Geometry check sheet. Reference: the model listing, model coordinates, mm. Round coordinates to 2 decimals unless told otherwise and drop trailing zeros. Loops run counter-clockwise (first coordinate to the right, second up) from the corner with the lowest first, then second, coordinate; pieces in that order, holes last. Notation, with made-up numbers: (66.25, 53.5) - (122.25, 53.5) arc R12 ccw to (122.25, 71.5) - close; hole circle Ø4 at (87.25, -37). An arc over 180 degrees is marked (long way). Answer as CSV lines item,"result". Start each with the question number.
1) Cross-section at D-D on y = -132. Record the boundary of the cut face in (x, z), and give its area (3 significant figures).
2) Thickness scan on line 1 along X through (y, z) = (-152, -1); line 2 along X through (y, z) = (-31.5, -1.75); line 3 along X through (y, z) = (-23, 1). Record the ranges inside material, lowest first.
3) Cross-section at A-A on y = -152. Record the boundary of the cut face in (x, z).
4) Depth check by flat-ended pin: P1, Ø1.5, axis at x = 1, y = -61.5, coming from the +Z side; P2, Ø3, axis at x = 7, y = -56, coming from the +Z side. Enter the tip coordinate at first touch or a pass-through.
5) Cross-section at B-B on z = -0.75. State how many separate pieces and enclosed holes the cut face has, and give its area (3 significant figures).
from build123d import *

# Parameters (mm, degrees)
BASE_DEPTH  = 160
ESQUISSE2_R = 2.5
TROU_DEPTH  = 161.624562256


with BuildPart() as part:
    # Esquisse1 → BASE (new body)
    with BuildSketch(Plane(origin=(0, 0, 0), x_dir=(1, 0, 0), z_dir=(0, 1, 0))):
        Polygon((-2, -3.75), (-2, 2.75), (2, 2.75), (2, -3.75), (12, -3.75), (12, 3.75), (-12, 3.75), (-12, -3.75), align=None)
    extrude(amount=-BASE_DEPTH)

    # Esquisse2 → TROU (cut, through all)
    with BuildSketch(Plane.XY.offset(3.75)):
        with Locations((-7, -8)):
            Circle(ESQUISSE2_R)
        with Locations((7, -8)):
            Circle(ESQUISSE2_R)
        with Locations((7, -24)):
            Circle(ESQUISSE2_R)
        with Locations((7, -40)):
            Circle(ESQUISSE2_R)
        with Locations((7, -56)):
            Circle(ESQUISSE2_R)
        with Locations((7, -72)):
            Circle(ESQUISSE2_R)
        with Locations((7, -88)):
            Circle(ESQUISSE2_R)
        with Locations((7, -104)):
            Circle(ESQUISSE2_R)
        with Locations((7, -120)):
            Circle(ESQUISSE2_R)
        with Locations((7, -136)):
            Circle(ESQUISSE2_R)
        with Locations((7, -152)):
            Circle(ESQUISSE2_R)
        with Locations((-7, -24)):
            Circle(ESQUISSE2_R)
        with Locations((-7, -40)):
            Circle(ESQUISSE2_R)
        with Locations((-7, -56)):
            Circle(ESQUISSE2_R)
        with Locations((-7, -72)):
            Circle(ESQUISSE2_R)
        with Locations((-7, -88)):
            Circle(ESQUISSE2_R)
        with Locations((-7, -104)):
            Circle(ESQUISSE2_R)
        with Locations((-7, -120)):
            Circle(ESQUISSE2_R)
        with Locations((-7, -136)):
            Circle(ESQUISSE2_R)
        with Locations((-7, -152)):
            Circle(ESQUISSE2_R)
    extrude(amount=-TROU_DEPTH, mode=Mode.SUBTRACT)


solid = part.part
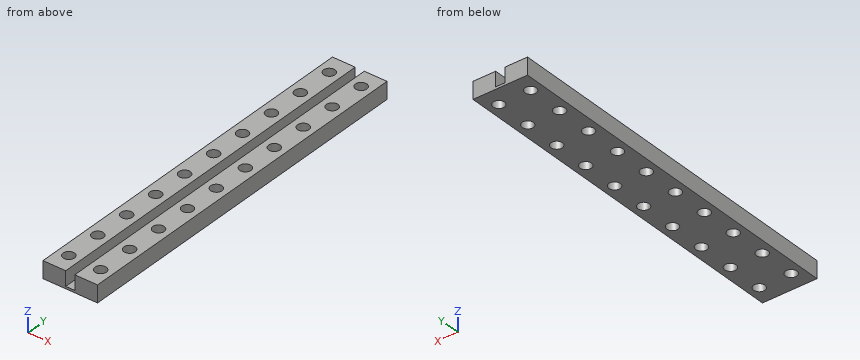
Answer block:
1,outline,"(-12, -3.75) - (12, -3.75) - (12, 3.75) - (2, 3.75) - (2, -2.75) - (-2, -2.75) - (-2, 3.75) - (-12, 3.75) - close"
1,area,"154 mm^2"
2,line 1,"x = -12 to -9.5, -4.5 to -2, 2 to 4.5, 9.5 to 12"
2,line 2,"x = -12 to -2, 2 to 12"
2,line 3,"x = -12 to -9.29, -4.71 to -2, 2 to 4.71, 9.29 to 12"
3,outline,"(-12, -3.75) - (-9.5, -3.75) - (-9.5, 3.75) - (-12, 3.75) - close; (-4.5, -3.75) - (4.5, -3.75) - (4.5, 3.75) - (2, 3.75) - (2, -2.75) - (-2, -2.75) - (-2, 3.75) - (-4.5, 3.75) - close; (9.5, -3.75) - (12, -3.75) - (12, 3.75) - (9.5, 3.75) - close"
4,P1,"stops at z = -2.75"
4,P2,"passes through"
5,separate pieces,"2"
5,enclosed holes,"20"
5,area,"2,810 mm^2"
